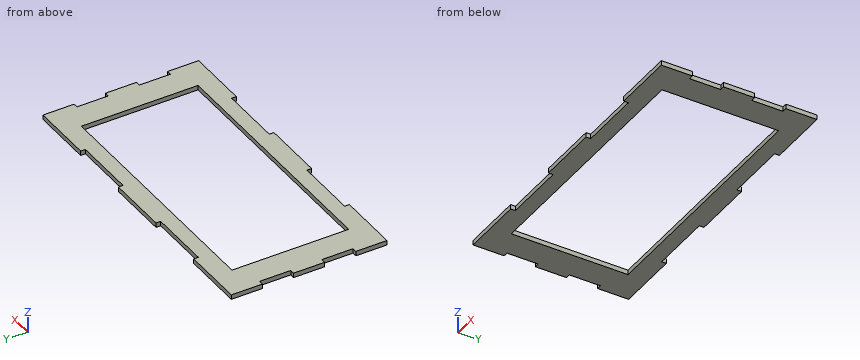
```python
from build123d import *

# Parameters (mm, degrees)
F1_DEPTH = 3


with BuildPart() as f1:
    # F0 (on Top) → F1 (new body)
    with BuildSketch(Plane.XY):
        Polygon((0, -20), (0, 0), (-40, 0), (-40, -3), (-80, -3), (-80, 0), (-120, 0), (-120, -3), (-160, -3), (-160, 0), (-200, 0), (-200, -20), (-197, -20), (-197, -40), (-200, -40), (-200, -60), (-197, -60), (-197, -80), (-200, -80), (-200, -100), (-160, -100), (-160, -97), (-120, -97), (-120, -100), (-80, -100), (-80, -97), (-40, -97), (-40, -100), (0, -100), (0, -80), (-3, -80), (-3, -60), (0, -60), (0, -40), (-3, -40), (-3, -20), align=None)
        Polygon((-180, -12.5), (-100, -12.5), (-20, -12.5), (-20, -87.5), (-180, -87.5), align=None, mode=Mode.SUBTRACT)
    extrude(amount=F1_DEPTH)


solid = f1.part
```
Geometry check sheet. Reference: the model listing, model coordinates, mm. Coordinates: 2 decimals unless noted, no trailing zeros. Write each loop counter-clockwise with the first axis right and the second up, starting at its lowest first coordinate (ties: lowest second). Pieces come first, ordered by that corner, then holes. Notation, with made-up numbers: M 11,2 L 27,2 A23 cw 27,41 Z; hole C 11.25,-37 d2. An arc over 180 degrees is marked long. Use one line per item in the form item = value. Start each with the question number.
1) Section check A-A on x = -133. Enter the section's corners in (y, z).
2) Thickness scan on probe 1 along X at (y, z) = (-63, 2.3); probe 2 along Y at (x, z) = (-59, 2.5); probe 3 along X at (y, z) = (-19, 2.6). Record the ranges inside material, lowest first. Write a range as from..to.
3) Go/stop test with flat-tipped pins: pin 1 Ø1.5 at (x, z) = (-130.5, 1.5) entering from -Y; pin 2 Ø1.5 at (y, z) = (-27.5, 2.5) entering from +X; pin 3 Ø1.5 at (y, z) = (-1, 2) entering from +X; pin 4 Ø0.9 at (x, z) = (-69, 1.5) entering from +Y. Record where each tip stops, or that it passes through.
4) Section check B-B on y = -78. Enter the section's corners in (x, z).
Responses:
q1.outline = M -97,0 L -87.5,0 L -87.5,3 L -97,3 Z; M -12.5,0 L -3,0 L -3,3 L -12.5,3 Z
q2.probe_1 = -197..-180, -20..-3
q2.probe_2 = -97..-87.5, -12.5..-3
q2.probe_3 = -200..-180, -20..0
q3.pin_1 = -97
q3.pin_2 = -3
q3.pin_3 = 0
q3.pin_4 = -3
q4.outline = M -197,0 L -180,0 L -180,3 L -197,3 Z; M -20,0 L -3,0 L -3,3 L -20,3 Z
